The listing builds one solid part. Answer for the finished solid, in the listing's coordinates (mm). A direction names the side the tool comes from. Round coordinates to 2 decimals unless told otherwise and drop trailing zeros. Order: outer loops, then holes, each group sorted by start corner. A loop starts at its lowest first (then second) coordinate and runs counter-clockwise, first axis right, second up. Notation, with made-up numbers: M 66.5,70 L 79.5,70 A23 cw 79.5,87 Z; hole C -14.5,25.5 d3. An arc over 180 degrees is marked long. Put each result on its own line as item: value. Start each with the question number.
1. The part is cut by section D-D (z = -22.5). Give the vertices of the cut face in (x, y) (3 decimals), then the cut area to 3 significant figures.
2. Which of the six approach directions +Z, -Z, +X, -X, +Y, -Y give full straight-line access (tool end or side, diameter ignored) to faces 4 (the face through (23.498, -37, -24)), 5 (the face through (57.19, -15, 0.22)), 6 (the face through (52.2, -16.7, -1.7)), 7 (the face through (-14.602, -29, 0)), 8 (the face through (39, -28.575, 20))?
3. The part is cut by section B-B (z = 0). Count the separate pieces of the cut face and the enclosed holes in it, then the cut area to 3 significant figures.
4. Consider line 1 (Y direction, x = 0, z = 13.25); line 2 (X direction, y = -7, z = -10); line 3 (X direction, y = 2, z = -11). Determine where each line is inside the solid, lowest interval first.
5. Each of these flat-tipped pins is pushed along its axis until it touches: pin 1 Ø8 at (y, z) = (11, 8.5) entering from +X; pin 2 Ø10 at (x, z) = (-16.5, 12) entering from +Y; pin 3 Ø8 at (x, z) = (35.5, -25) entering from +Y (3 decimals); pin 4 Ø23 at (x, y) = (0, 0) entering from -Z. Where does it stop, or does it pass through?
6. The mould has two halves that part along Y. Classify faces 1 (the face through (39, -28.575, -20)), 2 (the face through (94.79, -8.57, -6.22)), 3 (the face through (-15, 17, -4.762)): +Y half, -Y half, draft (parallel to the pull), parting line (faces both ways), or undercut.
from build123d import *

# Parameters (mm, degrees)
SKETCH1_R               = 20.6375
SKETCH1_R_2             = 14.2875
SKETCH1_W               = 41.275
SKETCH1_H               = 15.875
BOSS_EXTRUDE1_DEPTH     = 4.7625
SKETCH1_5_R             = 20.6375
SKETCH1_5_R_2           = 14.2875
BOSS_EXTRUDE2_DEPTH     = 19.05
SKETCH1_6_W             = 41.275
SKETCH1_6_H             = 15.875
BOSS_EXTRUDE3_DEPTH     = 15.875
SKETCH1_7_W             = 41.275
SKETCH1_7_H             = 15.875
BOSS_EXTRUDE4_DEPTH     = 31.75
CUT_EXTRUDE1_START      = -28.575
CUT_EXTRUDE1_OUTLINE_R  = 6.35
CUT_EXTRUDE1_DEPTH      = 47.625
CUT_EXTRUDE4_START      = -1.5875
SKETCH2_5_R             = 12.7
SKETCH2_5_R_2           = 6.35
CUT_EXTRUDE4_DEPTH      = 1.5875
CUT_EXTRUDE5_DEPTH      = 122.144687625
CUT_EXTRUDE5_DEPTH_BACK = 122.144687625
SKETCH3_R               = 3.175
SKETCH4_R               = 3.175
CUT_EXTRUDE6_DEPTH      = 121.173461332
CUT_EXTRUDE7_REACH      = 130.416
CUT_EXTRUDE7_END_RADIUS = 14.2875
SKETCH5_R               = 1.984375


# Read off the part's stored shape, not the designer's step: Cut-Extrude1
with BuildPart() as part:
    # Sketch1 → Boss-Extrude1 (new, symmetric)
    # profile 1 of 5: a face of its own
    with BuildSketch(Plane.XY):
        with BuildLine():
            ThreePointArc((25.250733281, -15.875), (20.027995944, -13.136857515), (19.309384274, -7.283823529))
            ThreePointArc((19.309384274, -7.283823529), (4.342837348, -20.175385251), (-14.60235654, -14.583469742))
            Line((-14.60235654, -14.583469742), (-14.60235654, -44.45))
            Line((-14.60235654, -44.45), (23.49764346, -44.45))
            Line((23.49764346, -44.45), (23.49764346, -28.575))
            Line((23.49764346, -28.575), (64.77264346, -28.575))
            Line((64.77264346, -28.575), (64.77264346, -44.45))
            Line((64.77264346, -44.45), (106.04764346, -44.45))
            Line((106.04764346, -44.45), (106.04764346, 3.175))
            Line((106.04764346, 3.175), (68.639696837, 3.175))
            Line((68.639696837, 3.175), (59.474261314, -12.7))
            ThreePointArc((59.474261314, -12.7), (57.15, -15.024261314), (53.975, -15.875))
            Line((53.975, -15.875), (25.250733281, -15.875))
        make_face()
    # profile 2 of 5: a face of its own
    with BuildSketch(Plane.XY):
        Circle(SKETCH1_R)
        with Locations(Location((0, 0, 0), (0, 0, 180))):
            Circle(SKETCH1_R_2, mode=Mode.SUBTRACT)
    # profile 3 of 5: a face of its own
    with BuildSketch(Plane.XY):
        with BuildLine():
            ThreePointArc((-14.60235654, -14.583469742), (-20.24645141, -3.998451143), (-19.05, 7.9375))
            Line((-19.05, 7.9375), (-47.625, 7.9375))
            Line((-47.625, 7.9375), (-47.625, -6.35))
            Line((-47.625, -6.35), (-14.60235654, -14.583469742))
        make_face()
    # profile 4 of 5: a face of its own
    with BuildSketch(Plane.XY):
        with Locations((44.13514346, -36.5125)):
            Rectangle(SKETCH1_W, SKETCH1_H)
    # profile 5 of 5: a face of its own
    with BuildSketch(Plane.XY):
        with BuildLine():
            ThreePointArc((-19.05, 7.9375), (-11.4476253, 17.171437949), (0, 20.6375))
            Line((0, 20.6375), (-19.05, 20.6375))
            Line((-19.05, 20.6375), (-19.05, 7.9375))
        make_face()
    extrude(amount=BOSS_EXTRUDE1_DEPTH, both=True)

    # Sketch1<5> → Boss-Extrude2 (add, symmetric)
    with BuildSketch(Plane.XY):
        Circle(SKETCH1_5_R)
        with Locations(Location((0, 0, 0), (0, 0, 180))):
            Circle(SKETCH1_5_R_2, mode=Mode.SUBTRACT)
    extrude(amount=BOSS_EXTRUDE2_DEPTH, both=True)

    # Sketch1<6> → Boss-Extrude3 (add, symmetric)
    with BuildSketch(Plane.XY):
        with BuildLine():
            ThreePointArc((25.250733281, -15.875), (20.027995944, -13.136857515), (19.309384274, -7.283823529))
            ThreePointArc((19.309384274, -7.283823529), (4.342837348, -20.175385251), (-14.60235654, -14.583469742))
            Line((-14.60235654, -14.583469742), (-14.60235654, -44.45))
            Line((-14.60235654, -44.45), (23.49764346, -44.45))
            Line((23.49764346, -44.45), (23.49764346, -28.575))
            Line((23.49764346, -28.575), (64.77264346, -28.575))
            Line((64.77264346, -28.575), (64.77264346, -44.45))
            Line((64.77264346, -44.45), (106.04764346, -44.45))
            Line((106.04764346, -44.45), (106.04764346, 3.175))
            Line((106.04764346, 3.175), (68.639696837, 3.175))
            Line((68.639696837, 3.175), (59.474261314, -12.7))
            ThreePointArc((59.474261314, -12.7), (57.15, -15.024261314), (53.975, -15.875))
            Line((53.975, -15.875), (25.250733281, -15.875))
        make_face()
        with Locations((44.13514346, -36.5125)):
            Rectangle(SKETCH1_6_W, SKETCH1_6_H)
    extrude(amount=BOSS_EXTRUDE3_DEPTH, both=True)

    # Sketch1<7> → Boss-Extrude4 (add, symmetric)
    with BuildSketch(Plane.XY):
        with Locations((44.13514346, -36.5125)):
            Rectangle(SKETCH1_7_W, SKETCH1_7_H)
    extrude(amount=BOSS_EXTRUDE4_DEPTH, both=True)

    # Cut-Extrude1 outline → Cut-Extrude1 (cut)
    with BuildSketch(Plane(origin=(0, -15.875, 0), x_dir=(1, 0, 0), z_dir=(0, 1, 0)).offset(CUT_EXTRUDE1_START)):
        with Locations((39.612866641, 0)):
            Circle(CUT_EXTRUDE1_OUTLINE_R)
        Polygon((71.12264346, -5.715), (71.12264346, -15.875), (106.04764346, -15.875), (106.04764346, -3.175), (77.47264346, -3.175), (77.47264346, -5.715), align=None)
        Polygon((64.77264346, -15.875), (48.89764346, -31.75), (64.77264346, -31.75), align=None)
        Polygon((64.77264346, 31.75), (48.89764346, 31.75), (64.77264346, 15.875), align=None)
    extrude(amount=CUT_EXTRUDE1_DEPTH, mode=Mode.SUBTRACT)

    # Sketch2<5> → Cut-Extrude4 (cut)
    # profile 1 of 4: a face of its own
    with BuildSketch(Plane(origin=(0, -15.875, 0), x_dir=(1, 0, 0), z_dir=(0, 1, 0)).offset(CUT_EXTRUDE4_START)):
        with Locations(Location((39.612866641, 0, 0), (0, 0, 270))):
            Circle(SKETCH2_5_R)
        with Locations(Location((39.612866641, 0, 0), (0, 0, 270))):
            Circle(SKETCH2_5_R_2, mode=Mode.SUBTRACT)
    # profile 2 of 4: a face of its own
    with BuildSketch(Plane(origin=(0, -15.875, 0), x_dir=(1, 0, 0), z_dir=(0, 1, 0)).offset(CUT_EXTRUDE4_START)):
        Polygon((48.89764346, -31.75), (64.77264346, -15.875), (64.77264346, -31.75), align=None)
    # profile 3 of 4: a face of its own
    with BuildSketch(Plane(origin=(0, -15.875, 0), x_dir=(1, 0, 0), z_dir=(0, 1, 0)).offset(CUT_EXTRUDE4_START)):
        Polygon((64.77264346, 31.75), (48.89764346, 31.75), (64.77264346, 15.875), align=None)
    # profile 4 of 4: a face of its own
    with BuildSketch(Plane(origin=(0, -15.875, 0), x_dir=(1, 0, 0), z_dir=(0, 1, 0)).offset(CUT_EXTRUDE4_START)):
        Polygon((106.04764346, -3.175), (77.47264346, -3.175), (77.47264346, -5.715), (71.12264346, -5.715), (71.12264346, -15.875), (106.04764346, -15.875), align=None)
    extrude(amount=CUT_EXTRUDE4_DEPTH, mode=Mode.SUBTRACT)

    # Sketch3 → Cut-Extrude5 (cut, two sides: drawn at the far end of the back side and taken through both)
    with BuildSketch(Plane(origin=(0, -28.575, 0), x_dir=(1, 0, 0), z_dir=(0, 1, 0)).offset(-CUT_EXTRUDE5_DEPTH_BACK)):
        with Locations(Location((39.612866641, 23.8125, 0), (0, 0, 270))):
            Circle(SKETCH3_R)
        with Locations(Location((39.612866641, -23.8125, 0), (0, 0, 270))):
            Circle(SKETCH3_R)
    extrude(amount=CUT_EXTRUDE5_DEPTH + CUT_EXTRUDE5_DEPTH_BACK, mode=Mode.SUBTRACT)

    # Sketch4 → Cut-Extrude6 (cut, through all)
    with BuildSketch(Plane.XY.offset(3.175)):
        with Locations((91.76014346, -9.525)):
            Circle(SKETCH4_R)
        with Locations((91.76014346, -31.75)):
            Circle(SKETCH4_R)
    extrude(amount=-CUT_EXTRUDE6_DEPTH, mode=Mode.SUBTRACT)

    # Cut-Extrude7: up to this cylinder (the profile starts outside it)
    cut_extrude7_end = Plane(origin=(0, 0, 0), z_dir=(0, 0, -1)) * Cylinder(CUT_EXTRUDE7_END_RADIUS, 290.407, mode=Mode.PRIVATE)
    # Sketch5 → Cut-Extrude7 (cut, up to the surface)
    with BuildSketch(Plane(origin=(0, 20.6375, 0), x_dir=(1, 0, 0), z_dir=(0, 1, 0)), mode=Mode.PRIVATE) as cut_extrude7_sk1:
        with Locations(Location((0, 0, 0), (0, 0, 180))):
            Circle(SKETCH5_R)
    cut_extrude7_tool1 = extrude(cut_extrude7_sk1.sketch, amount=-CUT_EXTRUDE7_REACH, mode=Mode.PRIVATE) - cut_extrude7_end
    add(cut_extrude7_tool1.solids().sort_by_distance((0, 20.6375, 0))[0], mode=Mode.SUBTRACT)


solid = part.part
Resolved:
1. outline: M 23.498,-44.45 L 36.722,-44.45 L 36.722,-28.575 L 23.498,-28.575 Z; M 42.504,-44.45 L 58.148,-44.45 L 58.148,-28.575 L 42.504,-28.575 Z
1. area: 458 mm2
2. face 4: -Z, -X, +Y, -Y
2. face 5: +Z, -Z, +Y
2. face 6: +Y
2. face 7: +Z, -Z, -X, -Y
2. face 8: +Z, +X, -X, +Y
3. separate pieces: 2
3. enclosed holes: 2
3. area: 5,000 mm2
4. line 1: -44.45 to -14.29, 14.29 to 20.64
4. line 2: -19.41 to -12.46, 12.46 to 19.41, 62.77 to 89.84, 93.68 to 106.05
4. line 3: -20.54 to -14.15, 14.15 to 20.54, 67.96 to 106.05
5. pin 1: x = 19.41
5. pin 2: y = 17.14
5. pin 3: y = -28.575
5. pin 4: through
6. face 1: +Y half
6. face 2: undercut
6. face 3: draft
